Could you check a few things on this model? Use its own coordinates, in mm. Give positions to 0.01 mm unless a question says otherwise; leave off trailing zeros. Loops run counter-clockwise (first coordinate to the right, second up) from the corner with the lowest first, then second, coordinate; pieces in that order, holes last. Notation, with made-up numbers: M 27.5,8 L 72.5,8 A32 cw 72.5,45 Z; hole C 44,17 d3. An arc over 180 degrees is marked long. Answer in a Markdown table with one row per item. Add a question column.
```python
from build123d import *

# Parameters (mm, degrees)
SKETCH_1_W      = 350
SKETCH_1_H      = 430
SKETCH_1_R      = 3.5
SKETCH_1_R_2    = 10
SKETCH_1_R_3    = 6
EXTRUDE_1_DEPTH = 20
FILLET_1_R      = 20


with BuildPart() as part:
    # Sketch 1 → Extrude 1 (new body)
    with BuildSketch(Plane.XY):
        with Locations((115, 0)):
            Rectangle(SKETCH_1_W, SKETCH_1_H)
        with Locations((-28, 185)):
            Circle(SKETCH_1_R, mode=Mode.SUBTRACT)
        with Locations((28, 185)):
            Circle(SKETCH_1_R, mode=Mode.SUBTRACT)
        with Locations((28, -185)):
            Circle(SKETCH_1_R, mode=Mode.SUBTRACT)
        with Locations((-28, -185)):
            Circle(SKETCH_1_R, mode=Mode.SUBTRACT)
        Circle(SKETCH_1_R_2, mode=Mode.SUBTRACT)
        with Locations((0, 45)):
            Circle(SKETCH_1_R_3, mode=Mode.SUBTRACT)
        with Locations((0, -45)):
            Circle(SKETCH_1_R_3, mode=Mode.SUBTRACT)
    extrude(amount=EXTRUDE_1_DEPTH)

    # Fillet 1
    fillet_1_edges = [part.edges().sort_by_distance(p)[0] for p in [
        (-60, -215, 10),
        (-60, 215, 10),
    ]]
    fillet(fillet_1_edges, radius=FILLET_1_R)


solid = part.part
```
Item 1: Suppose I cut it at A-A (y = -45). List the corners of the cut face in (x, z) for me.
Item 2: Suppose I cut it at B-B (x = 0). List the corners of the cut face in (y, z) for me, then the cut area to 3 significant figures.
Item 3: For P1, Ø6.5, axis at x = 28, y = 185, coming from the -Z side (3 decimals); P2, Ø15.5, axis at x = 0, y = 45, coming from the +Z side, each with a flat end and sliding along its axis, tell me the tip position at first contact or that it passes through.
Item 4: I need wall thicknesses on L1, parallel to X at y = 185, z = 11.25; L2, parallel to Y at x = 28, z = 6.5; L3, parallel to Y at x = 0, z = 5.75. Which ranges of each line are inside material? Lowest first, please.
Item 5: If we mould it in two halves opening along Y, with no side actions, what happens to faces 1 (the face through (-60, -3, 10)), 2 (the face through (-54.297, 208.986, 10.14)), 3 (the face through (-1.301, -50.857, 9.86))? For each: +Y half, -Y half, draft (parallel to the pull), parting line (faces both ways), or undercut.
Values found:
| question | item | result |
|---|---|---|
| 1 | outline | M -60,0 L -6,0 L -6,20 L -60,20 Z; M 6,0 L 290,0 L 290,20 L 6,20 Z |
| 2 | outline | M -215,0 L -51,0 L -51,20 L -215,20 Z; M -39,0 L -10,0 L -10,20 L -39,20 Z; M 10,0 L 39,0 L 39,20 L 10,20 Z; M 51,0 L 215,0 L 215,20 L 51,20 Z |
| 2 | area | 7,720 mm² |
| 3 | P1 | through |
| 3 | P2 | z = 20 |
| 4 | L1 | -60 to -31.5, -24.5 to 24.5, 31.5 to 290 |
| 4 | L2 | -215 to -188.5, -181.5 to 181.5, 188.5 to 215 |
| 4 | L3 | -215 to -51, -39 to -10, 10 to 39, 51 to 215 |
| 5 | face 1 | draft |
| 5 | face 2 | +Y half |
| 5 | face 3 | undercut |
